The model under review builds one solid part; all positions refer to its coordinate system, in mm. A direction names the side the tool comes from. Give positions to 0.01 mm unless a question says otherwise; leave off trailing zeros. Order: outer loops, then holes, each group sorted by start corner. A loop starts at its lowest first (then second) coordinate and runs counter-clockwise, first axis right, second up. Notation, with made-up numbers: M 74.25,36 L 116.25,36 A21 cw 116.25,56 Z; hole C 54,52 d2. An arc over 180 degrees is marked long. One line per question, with ' | ' between items. Start each with the question number.
1. We need section A-A on z = 27. Write out the cut boundary in (x, y).
2. Wall thickness on L1, parallel to Y at x = -40.5, z = 36.5; L2, parallel to X at y = -12.5, z = 6.5; L3, parallel to Z at x = -25, y = -11: over which ranges is each line inside the solid? List them lowest first.
3. For faces 4 (the face through (-51.6, -31.64, 30.07)), 5 (the face through (3, -27.5, 59)), 6 (the face through (51.64, -31.6, 30.93)), 7 (the face through (-49.5, 0, 57)), 8 (the face through (47.5, 0, 30)), list the 3-axis set-ups (+Z, -Z, +X, -X, +Y, -Y) from which the entire face can be reached by the end or side of a thin tool; tool diameter is ignored.
4. We need section B-B on y = 21. Write out the cut boundary in (x, z), then the cut area to 3 significant figures.
5. Insertion check: P1, Ø1.5, axis at y = 11.5, z = 59, coming from the +X side; P2, Ø1.5, axis at y = -0.5, z = 56.5, coming from the +X side; P3, Ø17.5, axis at x = 13.5, y = 4, coming from the +Z side. Each pin has a flat end and moves straight along its axis. Give the tip position at first contact, or say it passes through.
6. The part is to be moulded in two halves that separate along X. For faces 1 (the face through (-8, -29, 61)), 2 (the face through (-1, 0, 5)), 3 (the face through (-51.6, 31.64, 30.07)), say which applies: +X half, -X half, draft (parallel to the pull), parting line (faces both ways), or undercut.
7. We need section D-D on x = -36.5. Write out the cut boundary in (y, z).
```python
from build123d import *

# Parameters (mm, degrees)
F0_W      = 105
F0_H      = 65
F0_W_2    = 95
F0_H_2    = 55
F1_DEPTH  = 60
F2_DEPTH  = 5
F3_W      = 5
F3_H      = 55
F4_DEPTH  = 5
F6_DEPTH  = 2
F8_DEPTH  = 2
F10_DEPTH = 2
F11_R     = 2.99999
F12_R     = 1.5
F13_DEPTH = 1


# Not quite as in the source:
# - a fillet or chamfer is up to 0.001 mm smaller than in the source, because OpenCascade refuses the exact size


with BuildPart() as f1:
    # F0 (on Top) → F1 (new body)
    with BuildSketch(Plane.XY):
        Rectangle(F0_W, F0_H)
        Rectangle(F0_W_2, F0_H_2, mode=Mode.SUBTRACT)
    extrude(amount=F1_DEPTH)

    # F0 (on Top) → F2 (join)
    with BuildSketch(Plane.XY):
        Rectangle(F0_W_2, F0_H_2)
    extrude(amount=F2_DEPTH)

    # F3 (on face) → F4 (cut)
    with BuildSketch(Plane.XY.offset(60)):
        with Locations((50, 0)):
            Rectangle(F3_W, F3_H)
    extrude(amount=-F4_DEPTH, mode=Mode.SUBTRACT)

    # F5 (on face) → F6 (cut)
    with BuildSketch(Plane.XZ.offset(-27.5)):
        Polygon((47.5, 55), (52.5, 55), (52.5, 58), (-47.5, 58), (-47.5, 55), align=None)
    extrude(amount=-F6_DEPTH, mode=Mode.SUBTRACT)

    # F7 (on face) → F8 (cut)
    with BuildSketch(Plane.YZ.offset(-47.5)):
        Polygon((27.5, 55), (29.5, 55), (29.5, 58), (27.5, 58), (-27.5, 58), (-27.5, 55), align=None)
    extrude(amount=-F8_DEPTH, mode=Mode.SUBTRACT)

    # F9 (on face) → F10 (cut)
    with BuildSketch(Plane(origin=(0, -27.5, 0), x_dir=(-1, 0, 0), z_dir=(0, 1, 0))):
        Polygon((47.5, 55), (49.5, 55), (49.5, 58), (47.5, 58), (-52.5, 58), (-52.5, 55), (-47.5, 55), align=None)
    extrude(amount=-F10_DEPTH, mode=Mode.SUBTRACT)

    # F11 (radius 3 in the source; OpenCascade refuses exactly that, so slightly less here)
    f11_edges = [f1.edges().sort_by_distance(p)[0] for p in [
        (-52.5, -32.5, 30),
        (-52.5, 32.5, 30),
        (52.5, 32.5, 30),
        (52.5, -32.5, 30),
    ]]
    fillet(f11_edges, radius=F11_R)

    # F12
    f12_edges = [f1.edges().sort_by_distance(p)[0] for p in [
        (-49.5, -29.5, 56.5),
        (-49.5, 29.5, 56.5),
    ]]
    fillet(f12_edges, radius=F12_R)

    # F13 (add): a face of the model
    f13_faces = [f1.faces().sort_by_distance(p)[0] for p in [
        (-51.2650910965, 0, 60),
    ]]
    extrude(f13_faces, amount=F13_DEPTH)


solid = f1.part
```
Entries:
1) outline: M -52.5,-29.5 A3 ccw -49.5,-32.5 L 49.5,-32.5 A3 ccw 52.5,-29.5 L 52.5,29.5 A3 ccw 49.5,32.5 L -49.5,32.5 A3 ccw -52.5,29.5 Z; hole M -47.5,-27.5 L 47.5,-27.5 L 47.5,27.5 L -47.5,27.5 Z
2) L1: y = -32.5 to -27.5, 27.5 to 32.5 | L2: x = -52.5 to -47.5, 47.5 to 52.5 | L3: z = 0 to 5
3) face 4: +Z, -Z, -X, -Y | face 5: +Z, +X | face 6: +Z, -Z, +X, -Y | face 7: +X | face 8: +Z
4) outline: M -52.5,0 L 52.5,0 L 52.5,55 L 47.5,55 L 47.5,5 L -47.5,5 L -47.5,55 L -49.5,55 L -49.5,58 L -47.5,58 L -47.5,61 L -52.5,61 Z | area: 1,050 mm^2
5) P1: stops at x = -47.5 | P2: stops at x = -49.5 | P3: stops at z = 5
6) face 1: draft | face 2: undercut | face 3: -X half
7) outline: M -32.5,0 L 32.5,0 L 32.5,61 L 27.5,61 L 27.5,58 L 29.5,58 L 29.5,55 L 27.5,55 L 27.5,5 L -27.5,5 L -27.5,55 L -29.5,55 L -29.5,58 L -27.5,58 L -27.5,61 L -32.5,61 Z
